from build123d import *

# Parameters (mm, degrees)
SKETCH2_W                        = 1244.6
SKETCH2_H                        = 69.85
BASE_FLANGE1_DEPTH               = 3.2639
EDGE_FLANGE1_STRIP_W             = 15.5956
EDGE_FLANGE1_STRIP_H             = 3.2639
EDGE_FLANGE1_STRIP_CUT_DEPTH     = 1244.6
EDGE_FLANGE1_STRIP_2_W           = 15.5956
EDGE_FLANGE1_STRIP_2_H           = 3.2639
EDGE_FLANGE1_STRIP_CUT_2_DEPTH   = 1244.6
EDGE_FLANGE1_DEPTH               = 1244.6
EDGE_FLANGE1_BEND_DEPTH          = 1244.6
F_10_0_1935_DIAMETER_HOLE1_D     = 4.9149
SKETCH28_R                       = 21.87575
CUT_EXTRUDE1_DEPTH               = 631.49549328
F_10_0_1935_DIAMETER_HOLE5_D     = 4.9149
F_10_0_1935_DIAMETER_HOLE6_D     = 4.9149
F_10_0_1935_DIAMETER_HOLE7_D     = 4.9149
F_25_64_0_39063_DIAMETER_HOLE1_D = 9.922002
F_25_64_0_39063_DIAMETER_HOLE2_D = 9.922002
F_10_0_1935_DIAMETER_HOLE9_D     = 4.9149
LPATTERN1_COUNT                  = 13
LPATTERN1_PITCH                  = 101.6
FILLET3_R                        = 6.35
F_10_0_1935_DIAMETER_HOLE10_D    = 4.9149
F_10_0_1935_DIAMETER_HOLE11_D    = 4.9149


# Sheet-metal steps are written as plain solids
with BuildPart() as part:
    # Sketch2 → Base-Flange1 (new body)
    with BuildSketch(Plane.XY):
        Rectangle(SKETCH2_W, SKETCH2_H)
    extrude(amount=-BASE_FLANGE1_DEPTH)

    # Edge-Flange1 strip (across the edge) → Edge-Flange1 strip cut (cut)
    with BuildSketch(Plane(origin=(622.3, 34.925, 0), x_dir=(0, -1, 0), z_dir=(-1, 0, 0))):
        with Locations((-6.5278, -1.63195)):
            Rectangle(EDGE_FLANGE1_STRIP_W, EDGE_FLANGE1_STRIP_H)
    extrude(amount=EDGE_FLANGE1_STRIP_CUT_DEPTH, mode=Mode.SUBTRACT)

    # Edge-Flange1 strip 2 (across the edge) → Edge-Flange1 strip cut 2 (cut)
    with BuildSketch(Plane(origin=(-622.3, -34.925, 0), x_dir=(0, 1, 0), z_dir=(1, 0, 0))):
        with Locations((-6.5278, -1.63195)):
            Rectangle(EDGE_FLANGE1_STRIP_2_W, EDGE_FLANGE1_STRIP_2_H)
    extrude(amount=EDGE_FLANGE1_STRIP_CUT_2_DEPTH, mode=Mode.SUBTRACT)

    # Edge-Flange1 section (across the edge) → Edge-Flange1 (add)
    with BuildSketch(Plane(origin=(622.3, 34.925, 0), x_dir=(0, -1, 0), z_dir=(-1, 0, 0))):
        with BuildLine():
            Line((-3.2639, 1.27), (-3.2639, 66.5861))
            Line((-3.2639, 66.5861), (0, 66.5861))
            Line((0, 66.5861), (0, 1.27))
            ThreePointArc((0, 1.27), (0.371974388, 0.371974388), (1.27, 0))
            Line((1.27, 0), (1.27, -3.2639))
            ThreePointArc((1.27, -3.2639), (-1.935951435, -1.935951435), (-3.2639, 1.27))
        make_face()
    extrude(amount=EDGE_FLANGE1_DEPTH)

    # Edge-Flange1 section 2 (across the edge) → Edge-Flange1 bend (add)
    with BuildSketch(Plane(origin=(-622.3, -34.925, 0), x_dir=(0, 1, 0), z_dir=(1, 0, 0))):
        with BuildLine():
            Line((-3.2639, 1.27), (-3.2639, 66.5861))
            Line((-3.2639, 66.5861), (0, 66.5861))
            Line((0, 66.5861), (0, 1.27))
            ThreePointArc((0, 1.27), (0.371974388, 0.371974388), (1.27, 0))
            Line((1.27, 0), (1.27, -3.2639))
            ThreePointArc((1.27, -3.2639), (-1.935951435, -1.935951435), (-3.2639, 1.27))
        make_face()
    extrude(amount=EDGE_FLANGE1_BEND_DEPTH)

    # #10 (0.1935) Diameter Hole1 (through all)
    with Locations(Plane(origin=(0, 0, -3.2639), x_dir=(-1, 0, 0), z_dir=(0, 0, -1))):
        with Locations((552.45, 22.225), (603.25, 22.225), (603.25, -22.225), (552.45, -22.225), (501.65, -22.225), (501.65, 22.225)):
            Hole(F_10_0_1935_DIAMETER_HOLE1_D / 2)

    # Sketch28 → Cut-Extrude1 (cut, through all)
    with BuildSketch(Plane.XZ.offset(38.1889)):
        with Locations(Location((576.2625, 34.8361, 0), (0, 0, 270))):
            Circle(SKETCH28_R)
    extrude(amount=-CUT_EXTRUDE1_DEPTH, mode=Mode.SUBTRACT)

    # #10 (0.1935) Diameter Hole5 (through all)
    with Locations(Plane(origin=(0, -38.1889, 0), x_dir=(-1, 0, 0), z_dir=(0, -1, 0))):
        with Locations((-173.38675, -58.6486), (-173.38675, -11.0236), (-268.63675, -58.6486), (-268.63675, -11.0236)):
            Hole(F_10_0_1935_DIAMETER_HOLE5_D / 2)

    # #10 (0.1935) Diameter Hole6 (through all)
    with Locations(Plane(origin=(0, 0, -3.2639), x_dir=(-1, 0, 0), z_dir=(0, 0, -1))):
        with Locations((-233.71175, 22.225), (-208.31175, 22.225), (-208.31175, -22.225), (-233.71175, -22.225)):
            Hole(F_10_0_1935_DIAMETER_HOLE6_D / 2)

    # #10 (0.1935) Diameter Hole7 (through all)
    with Locations(Plane(origin=(0, 0, -3.2639), x_dir=(-1, 0, 0), z_dir=(0, 0, -1))):
        with Locations((463.55, 0), (368.3, 0)):
            Hole(F_10_0_1935_DIAMETER_HOLE7_D / 2)

    # 25/64 (0.39063) Diameter Hole1 (through all)
    with Locations(Plane(origin=(0, 0, -3.2639), x_dir=(-1, 0, 0), z_dir=(0, 0, -1))):
        with Locations((44.41825, -20.6375), (44.41825, 20.6375)):
            Hole(F_25_64_0_39063_DIAMETER_HOLE1_D / 2)

    # 25/64 (0.39063) Diameter Hole2 (through all)
    with Locations(Plane(origin=(0, 38.1889, 0), x_dir=(1, 0, 0), z_dir=(0, 1, 0))):
        with Locations((75.05065, -14.1986), (75.05065, -55.4736)):
            Hole(F_25_64_0_39063_DIAMETER_HOLE2_D / 2)

    # #10 (0.1935) Diameter Hole9 (through all)
    with Locations(Plane(origin=(0, -38.1889, 0), x_dir=(-1, 0, 0), z_dir=(0, -1, 0))):
        with Locations((609.6, -57.0611)):
            f_10_0_1935_diameter_hole9 = Hole(F_10_0_1935_DIAMETER_HOLE9_D / 2)

    # LPattern1: #10 (0.1935) Diameter Hole9 ×13, 7 skipped
    with Locations(*[(i * LPATTERN1_PITCH, 0, 0) for i in range(1, LPATTERN1_COUNT) if i not in (1, 3, 5, 7, 8, 10, 12)]):
        add(f_10_0_1935_diameter_hole9, mode=Mode.SUBTRACT)

    # Fillet3
    fillet3_edges = [part.edges().sort_by_distance(p)[0] for p in [
        (622.3, 36.55695, 66.5861),
        (-622.3, 36.55695, 66.5861),
        (-622.3, -36.55695, 66.5861),
        (622.3, -36.55695, 66.5861),
    ]]
    fillet(fillet3_edges, radius=FILLET3_R)

    # #10 (0.1935) Diameter Hole10 (through all)
    with Locations(Plane(origin=(0, 38.1889, 0), x_dir=(1, 0, 0), z_dir=(0, 1, 0))):
        with Locations((612.775, -12.6111), (612.775, -57.0611)):
            Hole(F_10_0_1935_DIAMETER_HOLE10_D / 2)

    # #10 (0.1935) Diameter Hole11 (through all)
    with Locations(Plane(origin=(0, 0, -3.2639), x_dir=(-1, 0, 0), z_dir=(0, 0, -1))):
        with Locations((-612.775, 19.05), (-612.775, -19.05)):
            Hole(F_10_0_1935_DIAMETER_HOLE11_D / 2)


solid = part.part
Can you work these out from the model? Positions are in its coordinate system, mm. A direction names the side the tool comes from. Round coordinates to 2 decimals unless told otherwise and drop trailing zeros. Order: outer loops, then holes, each group sorted by start corner. A loop starts at its lowest first (then second) coordinate and runs counter-clockwise, first axis right, second up. Notation, with made-up numbers: M 73.5,50.25 L 97.5,50.25 A23 cw 97.5,65.25 Z; hole C 25.5,56.5 d10. An arc over 180 degrees is marked long. Use a Markdown table: item, result.
1) Imagine slicing it at A-A (x = -132.5). List the corners of the cut face in (y, z) for me (3 decimals).
Geometry says:
| item | result |
|---|---|
| outline | M -38.189,1.27 A4.534 ccw -33.655,-3.264 L 33.655,-3.264 A4.534 ccw 38.189,1.27 L 38.189,66.586 L 34.925,66.586 L 34.925,1.27 A1.27 cw 33.655,0 L -33.655,0 A1.27 cw -34.925,1.27 L -34.925,66.586 L -38.189,66.586 Z |
2) Imagine slicing it at B-B (z = 38.5). List the corners of the cut face in (x, y) for me (3 decimals).
Geometry says:
| item | result |
|---|---|
| outline | M -622.3,-38.189 L 554.696,-38.189 L 554.696,-34.925 L -622.3,-34.925 Z; M -622.3,34.925 L 554.696,34.925 L 554.696,38.189 L -622.3,38.189 Z; M 597.829,-38.189 L 622.3,-38.189 L 622.3,-34.925 L 597.829,-34.925 Z; M 597.829,34.925 L 622.3,34.925 L 622.3,38.189 L 597.829,38.189 Z |
3) On a 3-axis mill with a long thin cutter (end or side, diameter ignored), from which of +Z, -Z, +X, -X, +Y, -Y can I reach the whole of each face in a straight line? I mean faces 4 (the face through (9, 34.925, 34)), 5 (the face through (9, 38.189, 33)). Say none if no direction works.
Geometry says:
| item | result |
|---|---|
| face 4 | +Z, +X, -X |
| face 5 | +Z, -Z, +X, -X, +Y |
4) If I drill on line 1 along Y through (x, z) = (255, 53.5) (3 decimals); line 2 along Z through (x, y) = (-355, -5), over which ranges is the centre line in solid material (lowest first)?
Geometry says:
| item | result |
|---|---|
| line 1 | y = -38.189 to -34.925, 34.925 to 38.189 |
| line 2 | z = -3.26 to 0 |
5) If we mould it in two halves opening along Y, with no side actions, what happens to faces 1 (the face through (-9, -38.189, 33)), 2 (the face through (-9, 0, 0)), 3 (the face through (622.3, 0, -2))? For each: +Y half, -Y half, draft (parallel to the pull), parting line (faces both ways), or undercut.
Geometry says:
| item | result |
|---|---|
| face 1 | -Y half |
| face 2 | undercut |
| face 3 | draft |
6) I'm going to push flat-ended pins straight in: P1, Ø6.5, axis at x = 233.71, y = 22.22, coming from the +Z side; P2, Ø4, axis at x = 612.78, z = 57.06, coming from the -Y side; P3, Ø16, axis at x = 75.05, z = 55.47, coming from the -Y side. Where does each tip first touch, or does it pass through?
Geometry says:
| item | result |
|---|---|
| P1 | stops at z = 0 |
| P2 | passes through |
| P3 | stops at y = -38.19 |
